```python
from build123d import *

# Parameters (mm, degrees)
F0_W     = 50
F0_H     = 40
F1_DEPTH = 30
F2_R     = 12
F3_DEPTH = 30.001
F4_D     = 3.2
F6_D     = 4.1


# Not quite as in the source:
# - a feature names something its author has since deleted; it is built from what else it names


with BuildPart() as f1:
    # F0 (on Front) → F1 (new body)
    with BuildSketch(Plane.XZ):
        with Locations((3.412880823, -1.3936108311)):
            Rectangle(F0_W, F0_H)
    extrude(amount=F1_DEPTH)

    # F2 (on face) → F3 (cut, through all)
    with BuildSketch(Plane.XZ.offset(30)):
        with Locations((3.412880823, -4.3936108311)):
            Circle(F2_R)
    extrude(amount=-F3_DEPTH, mode=Mode.SUBTRACT)

    # F4 (through all)
    with Locations(Plane.XZ.offset(30)):
        with Locations((-7.900827676, 6.9200976679), (-12.587119177, -4.3936108311), (-7.900827676, -15.7073193301), (14.726589322, -15.7073193301), (19.412880823, -4.3936108311), (14.726589322, 6.9200976679)):
            Hole(F4_D / 2)

    # F6 (through all)
    with Locations(Plane.XY.offset(18.6063891689)):
        with Locations((23.912880823, -22.5), (23.912880823, -7.5), (-17.087119177, -7.5), (-17.087119177, -22.5)):
            Hole(F6_D / 2)


solid = f1.part
```
Part model, mm, in its own coordinate system. Coordinates: 2 decimals unless noted, no trailing zeros. Loops run counter-clockwise (first coordinate to the right, second up) from the corner with the lowest first, then second, coordinate; pieces in that order, holes last. Notation, with made-up numbers: (-36, 33) - (-23, 33) arc R22 ccw to (-23, 64) - close; hole circle Ø2 at (28, -17.5). An arc over 180 degrees is marked (long way). Write item = value, one per line. Start each with the question number.
Item 1: Cut at B-B, the plane z = 4.5. Give the cut face in (x, y).
Item 2: Wall check: L1, parallel to X at y = -8.25, z = 13.5 (3 decimals); L2, parallel to X at y = -28.5, z = -15; L3, parallel to Z at x = -7, y = -3.5 (3 decimals). Give the ranges that are in metal, low to high. Write a range as from..to.
Item 3: Cut at A-A, the plane z = 14. Give the cut face in (x, y), and give its area (3 significant figures).
Item 4: Cut at D-D, the plane x = 23.5. Give the cut face in (y, z), and give its area (3 significant figures).
Item 5: Cut at C-C, the plane y = -7.5. State how many separate pieces and enclosed holes the cut face has, and give its area (3 significant figures).
Item 6: Mould opens along Y. For faces 1 (the flat face through (3, 0, 8)), 2 (the cylindrical face through (25.96, -7.41, -1.67)), 3 (the cylindrical face through (13.988, -14.79, -17.127)) say: released by +Y, released by -Y, zero draft, split by the parting line, or undercut.
The answers:
q1.outline = (-21.59, -30) - (-4.64, -30) - (-4.64, 0) - (-21.59, 0) - close; (11.47, -30) - (28.41, -30) - (28.41, 0) - (11.47, 0) - close; hole circle Ø4.1 at (-17.09, -22.5); hole circle Ø4.1 at (-17.09, -7.5); hole circle Ø4.1 at (23.91, -22.5); hole circle Ø4.1 at (23.91, -7.5)
q2.L1 = -21.587..-18.995, -15.179..22.005, 25.821..28.413
q2.L2 = -21.59..-9.34, -6.47..-2.2, 9.03..13.29, 16.16..28.41
q2.L3 = -21.394..-17.03, -14.385..-10.358, 1.571..5.598, 8.242..18.606
q3.outline = (-21.59, -30) - (28.41, -30) - (28.41, 0) - (-21.59, 0) - close; hole circle Ø4.1 at (-17.09, -22.5); hole circle Ø4.1 at (-17.09, -7.5); hole circle Ø4.1 at (23.91, -22.5); hole circle Ø4.1 at (23.91, -7.5)
q3.area = 1,450 mm2
q4.outline = (-30, -21.39) - (-24.51, -21.39) - (-24.51, 18.61) - (-30, 18.61) - close; (-20.49, -21.39) - (-9.51, -21.39) - (-9.51, 18.61) - (-20.49, 18.61) - close; (-5.49, -21.39) - (0, -21.39) - (0, 18.61) - (-5.49, 18.61) - close
q4.area = 879 mm2
q5.separate_pieces = 3
q5.enclosed_holes = 7
q5.area = 1,170 mm2
q6.face_1 = released by +Y
q6.face_2 = undercut
q6.face_3 = zero draft
